Geometry check sheet. Reference: drawing and pictorial views, mm from the part's lowest x, y, z. A direction names the side the tool comes from. Round coordinates to 2 decimals unless told otherwise and drop trailing zeros. Order: outer loops, then holes, each group sorted by start corner. A loop starts at its lowest first (then second) coordinate and runs counter-clockwise, first axis right, second up.
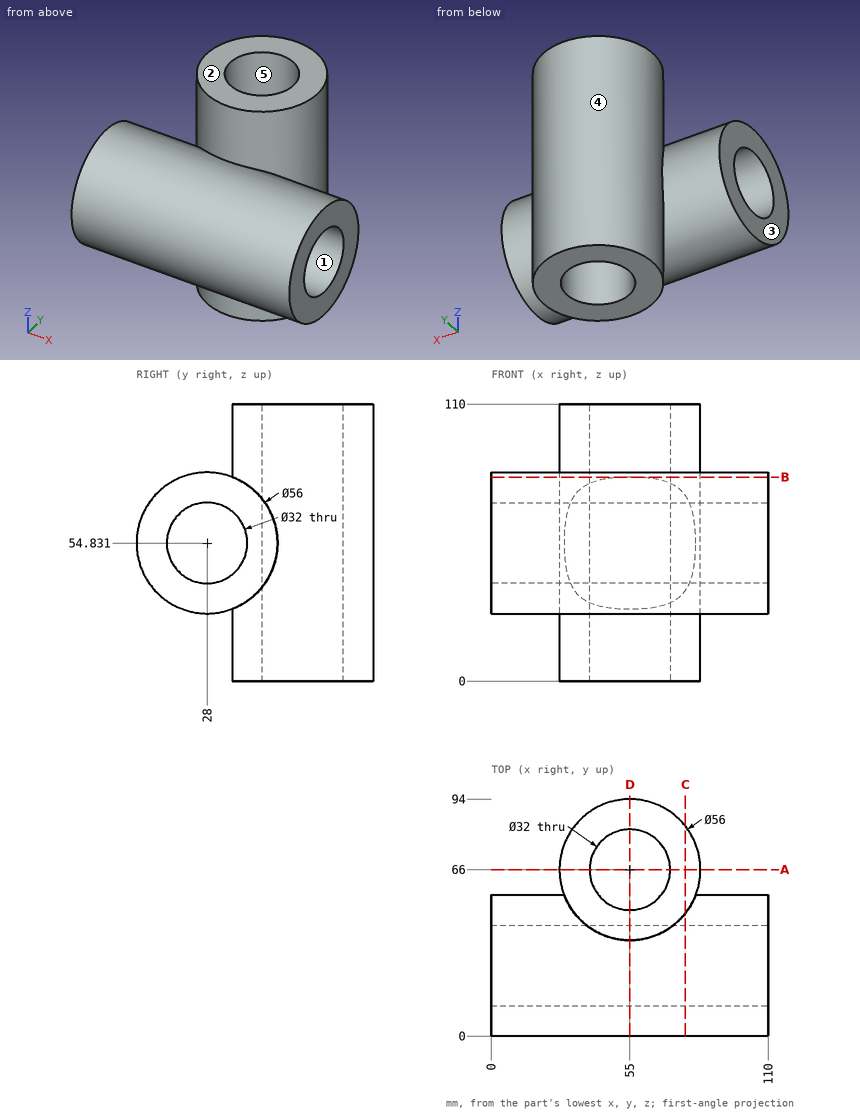
1) Sectioned sample at B-B on z = 81. Record the cut outline in (x, y), then the cut area to 3 significant figures.
2) Sectioned sample at D-D on x = 55. Record the cut outline in (y, z) (1 decimal).
3) Draft check along Z on the marked faces 1, 2 and 3. Enter one of: released by +Z, released by -Z, zero draft, split by the parting line, or undercut.
4) Sectioned sample at C-C on x = 77. Record the cut outline in (y, z).
5) Go/stop test with flat-tipped pins: pin 1 Ø6 at (x, z) = (54, 50.5) entering from +Y; pin 2 Ø8 at (y, z) = (66.5, 59) entering from +X; pin 3 Ø1.5 at (y, z) = (74, 98) entering from -X (1 decimal). Record where each tip stops, or that it passes through.
6) Sectioned sample at A-A on y = 66. Record the cut outline in (x, z).
7) Scan lines: probe 1 along Y at (x, z) = (55, 83); probe 2 along X at (y, z) = (52, 61) (1 decimal); probe 3 along Z at (x, y) = (35, 41) (1 decimal). Record each from-to range of solid material in increasing order.
8) Tool access check on the marked faces 4 and 5. Record the directions out of +Z, -Z, +X, -X, +Y, -Y that give a thin tool (end or side, any length) a straight path to the whole face; none if there is none.
Returned:
1. outline: (0, 18.04) - (110, 18.04) - (110, 37.96) - (0, 37.96) - close; circle Ø56 at (55, 66); hole circle Ø32 at (55, 66)
1. area: 3,850 mm2
2. outline: (38, 0) - (50, 0) - (50, 110) - (38, 110) - (38, 81) arc R28 ccw (long way) to (38, 28.7) - close; (82, 0) - (94, 0) - (94, 110) - (82, 110) - close; hole circle Ø32 at (28, 54.8)
3. face 1: undercut
3. face 2: released by +Z
3. face 3: zero draft
4. outline: (48.68, 0) - (83.32, 0) - (83.32, 110) - (48.68, 110) - (48.68, 73.71) arc R28 ccw (long way) to (48.68, 35.95) - close; hole circle Ø32 at (28, 54.83)
5. pin 1: stops at y = 94
5. pin 2: stops at x = 83
5. pin 3: stops at x = 28
6. outline: (27, 0) - (39, 0) - (39, 110) - (27, 110) - close; (71, 0) - (83, 0) - (83, 110) - (71, 110) - close
7. probe 1: y = 38 to 50, 82 to 94
7. probe 2: x = 0 to 47.3, 62.7 to 110
7. probe 3: z = 30 to 45.5, 64.2 to 79.6
8. face 4: none
8. face 5: +Z, -Z
